Geometry: final body of the model. Coordinates: model frame, mm. Round coordinates to 2 decimals unless told otherwise and drop trailing zeros. Order: outer loops, then holes, each group sorted by start corner. A loop starts at its lowest first (then second) coordinate and runs counter-clockwise, first axis right, second up. Notation, with made-up numbers: M 89,68.25 L 112,68.25 A27 ccw 112,104.25 Z; hole C -40,-2.75 d6. An arc over 180 degrees is marked long. Return JSON: item names as keys, results as strings. Group by question number.
Q1. Cut plane C-C on y = -7.75. Output: boundary loops of the cut face in (x, z), and give its area (3 significant figures).
Q2. Cut plane B-B on x = -29. Output: boundary loops of the cut face in (y, z).
Q3. Ray query, probe 1 along X at (y, z) = (1.5, 0.9); probe 2 along Y at (x, z) = (29, 0.8); probe 3 along Y at (x, z) = (25, 2.3). Return the intervals inside material, ascending.
Q4. Cut plane A-A on x = 25. Output: boundary loops of the cut face in (y, z).
Q5. Contact query for flat-ended pins moving along their axis: pin 1 (5 mm diameter, centred on x = 27.5, y = -1, fed in from -Z); pin 2 (5.5 mm diameter, centred on x = 25, y = 0, fed in from -Z). Output: stop coordinate, or through.
```python
from build123d import *

# Parameters (mm, degrees)
SKETCH1_R           = 3.5
BOSS_EXTRUDE1_DEPTH = 3


with BuildPart() as part:
    # Sketch1 → Boss-Extrude1 (new body)
    with BuildSketch(Plane.XY):
        with BuildLine():
            Line((-25, 9), (28.985507246, 6.5))
            add(Edge.make_bspline(
                [(28.985507246, 6.5), (40.946682853, 0), (28.985507246, -6.5)],
                knots=[0, 0, 0, 1, 1, 1], degree=2))
            Line((28.985507246, -6.5), (-25, -9))
            ThreePointArc((-25, -9), (-34, 0), (-25, 9))
        make_face()
        with Locations((25, 0)):
            Circle(SKETCH1_R, mode=Mode.SUBTRACT)
    extrude(amount=BOSS_EXTRUDE1_DEPTH)


solid = part.part
```
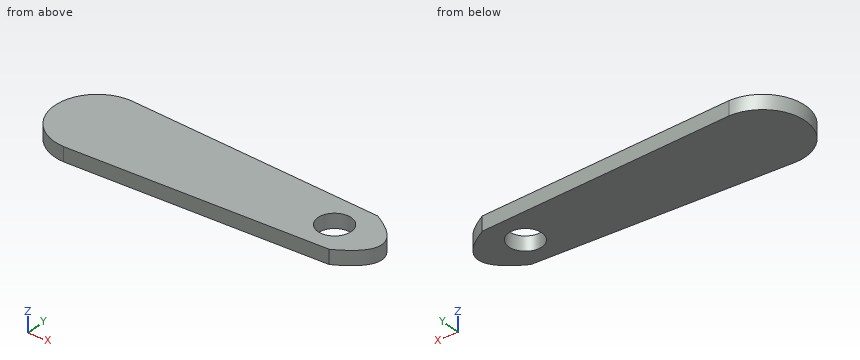
Result sheet:
{
 "1": {"outline": "M -29.58,0 L 1.99,0 L 1.99,3 L -29.58,3 Z", "area": "94.7 mm²"},
 "2": {"outline": "M -8.06,0 L 8.06,0 L 8.06,3 L -8.06,3 Z"},
 "3": {"probe 1": "x = -33.87 to 21.84, 28.16 to 34.65", "probe 2": "y = -6.49 to 6.49", "probe 3": "y = -6.68 to -3.5, 3.5 to 6.68"},
 "4": {"outline": "M -6.68,0 L -3.5,0 L -3.5,3 L -6.68,3 Z; M 3.5,0 L 6.68,0 L 6.68,3 L 3.5,3 Z"},
 "5": {"pin 1": "stops at z = 0", "pin 2": "passes through"}
}
